Here's how the part is built. I have some questions about the finished solid (model axes, mm). Face numbers are marked on the shaded views. A direction names the side the tool comes from. Round coordinates to 2 decimals unless told otherwise and drop trailing zeros. Loops run counter-clockwise (first coordinate to the right, second up) from the corner with the lowest first, then second, coordinate; pieces in that order, holes last. Notation, with made-up numbers: M 82.25,-3.5 L 131.25,-3.5 A21 cw 131.25,21.5 Z; hole C -18.75,68.25 d11. An arc over 180 degrees is marked long. Use a Markdown table: item, result.
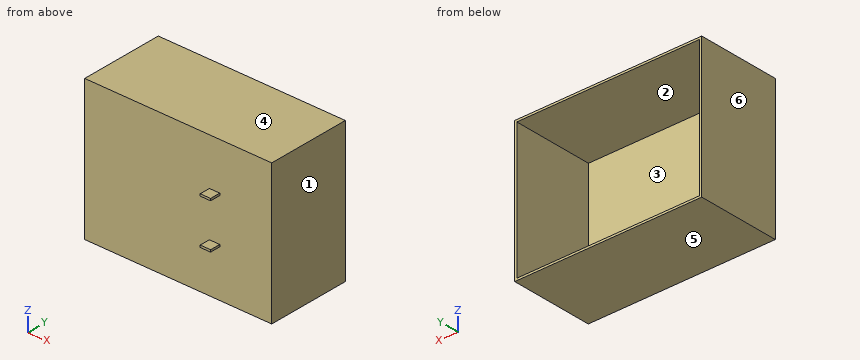
```python
from build123d import *

# Parameters (mm, degrees)
SKETCH1_W           = 900
SKETCH1_H           = 400
BOSS_EXTRUDE1_DEPTH = 675
SHELL1_T            = -10
SKETCH3_W           = 50
SKETCH3_H           = 10
BOSS_EXTRUDE4_DEPTH = 50


with BuildPart() as part:
    # Sketch1 → Boss-Extrude1 (new body)
    with BuildSketch(Plane.XY):
        with Locations((-450, 200)):
            Rectangle(SKETCH1_W, SKETCH1_H)
    extrude(amount=BOSS_EXTRUDE1_DEPTH)

    # Shell1
    shell1_openings = [part.faces().sort_by_distance(p)[0] for p in [
        (-450, 400, 337.5),
    ]]
    offset(amount=SHELL1_T, openings=shell1_openings, kind=Kind.INTERSECTION)

    # Sketch3 → Boss-Extrude4 (add)
    with BuildSketch(Plane(origin=(0, 0, 0), x_dir=(-1, 0, 0), z_dir=(0, -1, 0))):
        with Locations((275, -230)):
            Rectangle(SKETCH3_W, SKETCH3_H)
        with Locations((275, -445)):
            Rectangle(SKETCH3_W, SKETCH3_H)
    extrude(amount=BOSS_EXTRUDE4_DEPTH)


solid = part.part
```
Q1. I need wall thicknesses on line 1 (Z direction, x = -742, y = 294); line 2 (X direction, y = 186.5, z = 283); line 3 (Y direction, x = -840, z = 464). Which ranges of each line are inside material? Lowest first, please. Write a range as from..to.
Return value:
| item | result |
|---|---|
| line 1 | z = 0..10, 665..675 |
| line 2 | x = -900..-890, -10..0 |
| line 3 | y = 0..10 |
Q2. We'd pull the mould along Z, two halves only. Please class the marked faces 3, 4, 5 and 6: pulls with the +Z half, pulls with the -Z half, needs draft (parallel to the pull), parting line crosses it, or undercut.
Return value:
| item | result |
|---|---|
| face 3 | undercut |
| face 4 | pulls with the +Z half |
| face 5 | pulls with the -Z half |
| face 6 | needs draft |
Q3. For the marked faces 1 and 2, which set-ups out of +Z, -Z, +X, -X, +Y, -Y let a thin tool reach every point of the face, with its end or its side?
Return value:
| item | result |
|---|---|
| face 1 | +Z, -Z, +X, +Y, -Y |
| face 2 | +Y |
Q4. Imagine slicing it at B-B, the plane x = -690. Please give me the cut outline in (y, z).
Return value:
| item | result |
|---|---|
| outline | M 0,0 L 400,0 L 400,10 L 10,10 L 10,665 L 400,665 L 400,675 L 0,675 Z |
Q5. Imagine slicing it at C-C, the plane z = 83.5. Please give me the cut outline in (x, y).
Return value:
| item | result |
|---|---|
| outline | M -900,0 L 0,0 L 0,400 L -10,400 L -10,10 L -890,10 L -890,400 L -900,400 Z |
Q6. Imagine slicing it at A-A, the plane y = 304. Please give me the cut outline in (x, z), then the cut area to 3 significant figures.
Return value:
| item | result |
|---|---|
| outline | M -900,0 L 0,0 L 0,675 L -900,675 Z; hole M -890,10 L -10,10 L -10,665 L -890,665 Z |
| area | 31,100 mm^2 |
Q7. Will these pins go through, and if not, where does the flat tip stop? P1, Ø15, axis at x = -266.5, y = -34, coming from the +Z side; P2, Ø1.5, axis at x = -664.5, z = 127.5, coming from the -Y side; P3, Ø5, axis at y = -15, z = 443, coming from the -X side; P4, Ø4, axis at x = -727.5, y = 57.5, coming from the -Z side.
Return value:
| item | result |
|---|---|
| P1 | stops at z = 450 |
| P2 | stops at y = 0 |
| P3 | stops at x = -300 |
| P4 | stops at z = 0 |
